Source: CAD feature listing. Evaluate the final solid. Frame: model axes, mm. A direction names the side the tool comes from. Coordinates: 2 decimals unless noted, no trailing zeros. Loops run counter-clockwise (first coordinate to the right, second up) from the corner with the lowest first, then second, coordinate; pieces in that order, holes last.
Item 1: Section query A-A, the plane z = -19. Return the cut outline in (x, y), then the cut area to 3 significant figures.
Item 2: Section query C-C, the plane x = 30. Return the cut outline in (y, z), then the cut area to 3 significant figures.
Item 3: Reachability of faces 4 (the flat face through (1.2, 8, -19)), 5 (the flat face through (73.2, 1.2, -19.1)), 6 (the flat face through (0, 7, -19)) from +Z, -Z, +X, -X, +Y, -Y: full face, straight path, thin tool, end or side. Return the list, or none.
Item 4: Pull-direction query (Z, two-part tool) for faces 1 (the flat face through (32, 8, -36.8)), 2 (the flat face through (33, 7, -38)), 3 (the flat face through (23, 14, -37)); classes: +Z half, -Z half, draft (parallel to the pull), parting line (faces both ways), or undercut.
Item 5: Section query B-B, the plane y = 13.25. Return the cut outline in (x, z), then the cut area to 3 significant figures.
Item 6: Line query: probe 1 along Z at (x, y) = (30.5, 8.5); probe 2 along X at (y, z) = (9.25, -5); probe 3 along Y at (x, z) = (32.5, -23.5). Output: solid intervals per line, ascending.
Item 7: Pin query (flat end, axial travel): pin 1 Ø2 at (x, z) = (46, -10) entering from +Y; pin 2 Ø8 at (x, z) = (63, -10.5) entering from +Y; pin 3 Ø6.5 at (y, z) = (8.5, -15.5) entering from +X. Return the tip coordinate at first contact, or that it passes through.
```python
from build123d import *

# Parameters (mm, degrees)
SKETCH_1_W          = 75
SKETCH_1_H          = 38
EXTRUDE_1_DEPTH     = 14
SKETCH_2_W          = 10
SKETCH_2_H          = 38
CUT_EXTRUDE_1_DEPTH = 12.8
SKETCH_3_W          = 7
SKETCH_3_H          = 30
CUT_EXTRUDE_2_DEPTH = 1.2
FILLET_2_R          = 4
SKETCH_5_W          = 62.6
SKETCH_5_H          = 35.6
CUT_EXTRUDE_4_DEPTH = 12.8
FILLET_3_R          = 2
FILLET_4_R          = 2
FILLET_6_R          = 1
FILLET_7_R          = 1
FILLET_8_R          = 1


with BuildPart() as part:
    # Эскиз1 → Бобышка-Вытянуть1 (new body)
    with BuildSketch(Plane(origin=(0, 0, 0), x_dir=(1, 0, 0), z_dir=(0, 1, 0))):
        with Locations((37.5, 19)):
            Rectangle(SKETCH_1_W, SKETCH_1_H)
    extrude(amount=EXTRUDE_1_DEPTH)

    # Эскиз2 → Вырез-Вытянуть1 (cut)
    with BuildSketch(Plane(origin=(0, 14, 0), x_dir=(1, 0, 0), z_dir=(0, 1, 0))):
        with Locations((70, 19)):
            Rectangle(SKETCH_2_W, SKETCH_2_H)
    extrude(amount=-CUT_EXTRUDE_1_DEPTH, mode=Mode.SUBTRACT)

    # Эскиз3 → Вырез-Вытянуть2 (cut)
    with BuildSketch(Plane(origin=(0, 1.2, 0), x_dir=(1, 0, 0), z_dir=(0, 1, 0))):
        with Locations((68.5, 19)):
            Rectangle(SKETCH_3_W, SKETCH_3_H)
    extrude(amount=-CUT_EXTRUDE_2_DEPTH, mode=Mode.SUBTRACT)

    # Скругление2
    fillet_2_edges = [part.edges().sort_by_distance(p)[0] for p in [
        (75, 0.6, -38),
        (75, 0.6, 0),
        (72, 0.6, -34),
        (72, 0.6, -4),
    ]]
    fillet(fillet_2_edges, radius=FILLET_2_R)

    # Эскиз5 → Вырез-Вытянуть4 (cut)
    with BuildSketch(Plane(origin=(0, 14, 0), x_dir=(1, 0, 0), z_dir=(0, 1, 0))):
        with Locations((32.5, 19)):
            Rectangle(SKETCH_5_W, SKETCH_5_H)
    extrude(amount=-CUT_EXTRUDE_4_DEPTH, mode=Mode.SUBTRACT)

    # Скругление3
    fillet_3_edges = [part.edges().sort_by_distance(p)[0] for p in [
        (0, 7, -38),
        (0, 7, 0),
    ]]
    fillet(fillet_3_edges, radius=FILLET_3_R)

    # Скругление4
    fillet_4_edges = [part.edges().sort_by_distance(p)[0] for p in [
        (1.2, 7.6, -1.2),
        (1.2, 7.6, -36.8),
        (63.8, 7.6, -36.8),
        (63.8, 7.6, -1.2),
    ]]
    fillet(fillet_4_edges, radius=FILLET_4_R)

    # Скругление6
    fillet_6_edges = [part.edges().sort_by_distance(p)[0] for p in [
        (36.5, 0, -38),
        (75, 0, -19),
        (73.828427125, 0, -1.171572875),
        (73.828427125, 0, -36.828427125),
        (0, 0, -19),
        (36.5, 0, 0),
        (0.585786438, 0, -0.585786438),
        (0.585786438, 0, -37.414213562),
    ]]
    fillet(fillet_6_edges, radius=FILLET_6_R)

    # Скругление7
    fillet_7_edges = [part.edges().sort_by_distance(p)[0] for p in [
        (66.5, 1.2, -4),
        (72, 1.2, -19),
        (66.5, 1.2, -34),
        (70.828427125, 1.2, -5.171572875),
        (70.828427125, 1.2, -32.828427125),
    ]]
    fillet(fillet_7_edges, radius=FILLET_7_R)

    # Скругление8
    # the kernel refuses this fillet: 1 mm, written as the material it takes off along each edge
    with BuildSketch(Plane(origin=(71, 1.2, -38), x_dir=(0, 0, 1), z_dir=(-1, 0, 0)), Plane(origin=(65, 1.2, 0), x_dir=(0, 0, -1), z_dir=(1, 0, 0))) as fillet_8_piece_1:
        with BuildLine():
            CenterArc((0.6, -1), FILLET_8_R, 90, 36.869897646)
            Line((0, -0.2), (-0.012, -0.184))
            ThreePointArc((-0.012, -0.184), (-0.02, -0.1), (-0.02, 0))
            Line((-0.02, 0), (0, 0.02))
            Line((0, 0.02), (0.6, 0.02))
            Line((0.6, 0.02), (0.6, 0))
        make_face()
    extrude(amount=6, mode=Mode.SUBTRACT)
    with BuildSketch(Plane(origin=(71, 1.2, -34), x_dir=(1, 0, 0), z_dir=(0, 0, 1))) as fillet_8_piece_2:
        with BuildLine():
            CenterArc((3.4, -1), FILLET_8_R, 53.130102354, 36.869897646)
            Line((4, -0.2), (4.012, -0.184))
            ThreePointArc((4.012, -0.184), (4.02, -0.1), (4.02, 0))
            Line((4.02, 0), (4, 0.02))
            Line((4, 0.02), (3.4, 0.02))
            Line((3.4, 0.02), (3.4, 0))
        make_face()
    revolve(axis=Axis((71, 1.2, -34), (0, 1, 0)), revolution_arc=90, mode=Mode.SUBTRACT)
    with BuildSketch(Plane(origin=(75, 1.2, -4), x_dir=(-1, 0, 0), z_dir=(0, 0, -1))) as fillet_8_piece_3:
        with BuildLine():
            CenterArc((0.6, -1), FILLET_8_R, 90, 36.869897646)
            Line((0, -0.2), (-0.012, -0.184))
            ThreePointArc((-0.012, -0.184), (-0.02, -0.1), (-0.02, 0))
            Line((-0.02, 0), (0, 0.02))
            Line((0, 0.02), (0.6, 0.02))
            Line((0.6, 0.02), (0.6, 0))
        make_face()
    extrude(amount=30, mode=Mode.SUBTRACT)
    with BuildSketch(Plane(origin=(71, 1.2, -4), x_dir=(0, 0, 1), z_dir=(-1, 0, 0))) as fillet_8_piece_4:
        with BuildLine():
            CenterArc((3.4, -1), FILLET_8_R, 53.130102354, 36.869897646)
            Line((4, -0.2), (4.012, -0.184))
            ThreePointArc((4.012, -0.184), (4.02, -0.1), (4.02, 0))
            Line((4.02, 0), (4, 0.02))
            Line((4, 0.02), (3.4, 0.02))
            Line((3.4, 0.02), (3.4, 0))
        make_face()
    revolve(axis=Axis((71, 1.2, -4), (0, 1, 0)), revolution_arc=90, mode=Mode.SUBTRACT)


solid = part.part
```
Verdict:
1. outline: (0, 1) arc R1 ccw to (1, 0) - (65, 0) - (65, 14) - (63.8, 14) - (63.8, 1.2) - (1.2, 1.2) - (1.2, 14) - (0, 14) - close; (72, 0) - (74, 0) arc R1 ccw to (75, 1) arc R1 ccw to (74.4, 1.2) - (73, 1.2) arc R1 ccw to (72, 0.2) - close
1. area: 112 mm2
2. outline: (0, -37) arc R1 ccw to (1, -38) - (14, -38) - (14, -36.8) - (1.2, -36.8) - (1.2, -1.2) - (14, -1.2) - (14, 0) - (1, 0) arc R1 ccw to (0, -1) - close
2. area: 75.9 mm2
3. face 4: +Y
3. face 5: +Z, -Z, +X, +Y
3. face 6: +Z, -Z, -X, +Y, -Y
4. face 1: undercut
4. face 2: -Z half
4. face 3: draft
5. outline: (0, -36) arc R2 ccw to (2, -38) - (65, -38) - (65, 0) - (2, 0) arc R2 ccw to (0, -2) - close; hole (1.2, -34.8) arc R2 ccw to (3.2, -36.8) - (61.8, -36.8) arc R2 ccw to (63.8, -34.8) - (63.8, -3.2) arc R2 ccw to (61.8, -1.2) - (3.2, -1.2) arc R2 ccw to (1.2, -3.2) - close
5. area: 243 mm2
6. probe 1: z = -38 to -36.8, -1.2 to 0
6. probe 2: x = 0 to 1.2, 63.8 to 65
6. probe 3: y = 0 to 1.2
7. pin 1: stops at y = 1.2
7. pin 2: stops at y = 14
7. pin 3: stops at x = 65
